```python
from build123d import *

# Parameters (mm, degrees)
SKETCH1_R           = 5
BOSS_EXTRUDE1_DEPTH = 6


with BuildPart() as part:
    # Sketch1 → Boss-Extrude1 (new body)
    with BuildSketch(Plane(origin=(0, 0, 0), x_dir=(1, 0, 0), z_dir=(0, 1, 0))):
        Polygon((13.673278968, -16.635546923), (4.478237082, -16.635546923), (4.478237082, -4.635546923), (10.478237082, -4.635546923), (10.478237082, 7.364453077), (4.478237082, 7.364453077), (4.478237082, 19.364453077), (10.478237082, 19.364453077), (10.478237082, 29.311113477), (83.225400432, 29.311113477), (83.225400432, 19.364453077), (89.225400432, 19.364453077), (89.225400432, 7.364453077), (83.225400432, 7.364453077), (83.225400432, -4.635546923), (89.225400432, -4.635546923), (89.225400432, -16.635546923), (80.030358547, -16.635546923), (77.395115136, 0.405693798), (53.496778433, 0.405693798), (53.496778433, 20.432362651), (40.206859082, 20.432362651), (40.206859082, 0.405693798), (16.308522379, 0.405693798), align=None)
        with Locations(Location((28.974519722, 7.237839647, 0), (0, 0, 270))):
            Circle(SKETCH1_R, mode=Mode.SUBTRACT)
        with Locations(Location((64.729117792, 7.237839647, 0), (0, 0, 270))):
            Circle(SKETCH1_R, mode=Mode.SUBTRACT)
    extrude(amount=BOSS_EXTRUDE1_DEPTH)


solid = part.part
```
Here's how the part is built. I have some questions about the finished solid (model axes, mm). A direction names the side the tool comes from. Coordinates: 2 decimals unless noted, no trailing zeros. Order: outer loops, then holes, each group sorted by start corner. A loop starts at its lowest first (then second) coordinate and runs counter-clockwise, first axis right, second up. Notation, with made-up numbers: M 10,43 L 34,43 A11 ccw 34,49 Z; hole C 79,47.25 d1. An arc over 180 degrees is marked long. Answer as a JSON object with one key per item and string values. Group by question number.
(1) Suppose I cut it at A-A, the plane z = -15.5. Please give me the cut outline in (x, y), then the cut area to 3 significant figures.
(2) I need wall thicknesses on probe 1 along X at (y, z) = (3.95, -18.5); probe 2 along Z at (x, y) = (83.5, 1.3); probe 3 along X at (y, z) = (1.6, -3). Which ranges of each line are inside material? Lowest first, please.
(3) Suppose I cut it at D-D, the plane y = 3.45. Please give me the cut outline in (x, z).
(4) Suppose I cut it at B-B, the plane x = 67.5. Please give me the cut outline in (y, z), then the cut area to 3 significant figures.
(5) Which directions (+Z, -Z, +X, -X, +Y, -Y) give clear straight access to the entire face, cutting with the end or side of a thin tool? Please do faces 4 (the face through (83.225, 3, -1)), 5 (the face through (83.225, 3, -24)), 6 (the face through (15.01, 2.96, 8)), 7 (the face through (4.478, 3, -13)), 8 (the face through (10.478, 3, -24)).
(6) If we mould it in two halves opening along X, with no side actions, what happens to faces 1 (the face through (9, 3, 16.636)), 2 (the face through (47, 3, -20.432)), 3 (the face through (4.478, 3, 11))? For each: released by +X, released by -X, zero draft, split by the parting line, or undercut.
(7) For pin 1 (3 mm diameter, centred on y = 3.5, z = -26, fed in from -X); pin 2 (3 mm diameter, centred on x = 48.5, y = 5.5, fed in from +Z); pin 3 (8 mm diameter, centred on x = 28.97, z = -7.24, fed in from -Y); pin 4 (3 mm diameter, centred on x = 6, y = 2, fed in from -Z), each with a flat end and sliding along its axis, tell me the tip position at first contact or that it passes through.
(8) Suppose I cut it at C-C, the plane z = -10.5. Please give me the cut outline in (x, y).
Values found:
{
 "1": {"outline": "M 4.48,0 L 40.21,0 L 40.21,6 L 4.48,6 Z; M 53.5,0 L 89.23,0 L 89.23,6 L 53.5,6 Z", "area": "429 mm^2"},
 "2": {"probe 1": "x = 4.48 to 40.21, 53.5 to 89.23", "probe 2": "z = -19.36 to -7.36, 4.64 to 16.64", "probe 3": "x = 10.48 to 26.32, 31.63 to 40.21, 53.5 to 62.08, 67.38 to 83.23"},
 "3": {"outline": "M 4.48,-19.36 L 10.48,-19.36 L 10.48,-29.31 L 83.23,-29.31 L 83.23,-19.36 L 89.23,-19.36 L 89.23,-7.36 L 83.23,-7.36 L 83.23,4.64 L 89.23,4.64 L 89.23,16.64 L 80.03,16.64 L 77.4,-0.41 L 53.5,-0.41 L 53.5,-20.43 L 40.21,-20.43 L 40.21,-0.41 L 16.31,-0.41 L 13.67,16.64 L 4.48,16.64 L 4.48,4.64 L 10.48,4.64 L 10.48,-7.36 L 4.48,-7.36 Z; hole C 28.97,-7.24 d10; hole C 64.73,-7.24 d10"},
 "4": {"outline": "M 0,-29.31 L 6,-29.31 L 6,-11.4 L 0,-11.4 Z; M 0,-3.08 L 6,-3.08 L 6,-0.41 L 0,-0.41 Z", "area": "123 mm^2"},
 "5": {"face 4": "+X, +Y, -Y", "face 5": "-Z, +X, +Y, -Y", "face 6": "+Z, +Y, -Y", "face 7": "+Z, -Z, -X, +Y, -Y", "face 8": "-Z, -X, +Y, -Y"},
 "6": {"face 1": "zero draft", "face 2": "undercut", "face 3": "released by -X"},
 "7": {"pin 1": "stops at x = 10.48", "pin 2": "stops at z = -20.43", "pin 3": "passes through", "pin 4": "stops at z = -19.36"},
 "8": {"outline": "M 4.48,0 L 25.19,0 L 25.19,6 L 4.48,6 Z; M 32.76,0 L 40.21,0 L 40.21,6 L 32.76,6 Z; M 53.5,0 L 60.94,0 L 60.94,6 L 53.5,6 Z; M 68.52,0 L 89.23,0 L 89.23,6 L 68.52,6 Z"}
}
